Verification items for the finished model (mm, model axes). A direction names the side the tool comes from. Give positions to 0.01 mm unless a question says otherwise; leave off trailing zeros. Order: outer loops, then holes, each group sorted by start corner. A loop starts at its lowest first (then second) coordinate and runs counter-clockwise, first axis right, second up.
(1) Access from +Z, -Z, +X, -X, +Y, -Y to the whole of each face (thin tool, end or side, straight path). Record for faces 4 (the face through (-14.33, -0.37, 1.52)), 5 (the face through (-38.7, -39.23, 1.52)).
(2) Sectioned sample at B-B on x = -7.5. Record the cut outline in (y, z).
(3) Gauge pin test, flat ends, axial feed: pin 1 (4 mm diameter, centred on x = -7.5, y = -65, fed in from +Z); pin 2 (0.9 mm diameter, centred on x = -51.5, z = 1.5, fed in from -Y); pin 3 (1.5 mm diameter, centred on x = -29.5, z = 1, fed in from -Y); pin 4 (0.9 mm diameter, centred on y = -29.5, z = 1.5, fed in from -X). Record the tip position at first contact, or that the pin passes through.
(4) Sectioned sample at A-A on z = 2.45. Count the separate pieces of the cut face and the enclosed holes in it, plus the area to 3 significant figures.
(5) Mould release check, pull along X, two halves, no side actions. Record for faces 1 (the face through (-25.273, -5.418, 1.479)), 2 (the face through (-69, -2, 2)), 3 (the face through (0, -41, 1)): pulls with the +X half, pulls with the -X half, needs draft (parallel to the pull), parting line crosses it, or undercut.
(6) Scan lines: L1, parallel to X at y = -46, z = 1.85; L2, parallel to X at y = -25, z = 0.7; L3, parallel to X at y = -45, z = 1.25. Record each from-to range of solid material in increasing order.
```python
from build123d import *

# Parameters (mm, degrees)
SKETCH_1_R               = 2.1
EXTRUDE_1_DEPTH          = 3
EXTRUDE_2_DEPTH          = 3
CUT_EXTRUDE_1_DEPTH      = 100.040395799
CUT_EXTRUDE_1_DEPTH_BACK = 3
FILLET_1_R               = 5
EXTRUDE_3_DEPTH          = 3
FILLET_2_R               = 3
FILLET_3_R               = 10


with BuildPart() as part:
    # 草图1 → 凸台-拉伸1 (new body)
    with BuildSketch(Plane.XY):
        Polygon((0, 0), (-70, 0), (-70, -15), (-15, -15), (-15, -70), (0, -70), align=None)
        with Locations((-25, -7.5)):
            Circle(SKETCH_1_R, mode=Mode.SUBTRACT)
        with Locations(Location((-7.5, -25, 0), (0, 0, 180))):
            Circle(SKETCH_1_R, mode=Mode.SUBTRACT)
        with Locations((-45, -7.5)):
            Circle(SKETCH_1_R, mode=Mode.SUBTRACT)
        with Locations((-65, -7.5)):
            Circle(SKETCH_1_R, mode=Mode.SUBTRACT)
        with Locations(Location((-7.5, -65, 0), (0, 0, 180))):
            Circle(SKETCH_1_R, mode=Mode.SUBTRACT)
        with Locations(Location((-7.5, -45, 0), (0, 0, 180))):
            Circle(SKETCH_1_R, mode=Mode.SUBTRACT)
    extrude(amount=EXTRUDE_1_DEPTH)

    # 草图2 → 凸台-拉伸2 (add)
    with BuildSketch(Plane.XY.offset(3)):
        Polygon((-70, -15), (-15, -70), (-15, -62.928932188), (-62.928932188, -15), align=None)
    extrude(amount=-EXTRUDE_2_DEPTH)

    # 草图3 → 切除-拉伸1 (cut, two sides: drawn at the far end of the back side and taken through both)
    with BuildSketch(Plane.XY.offset(3).offset(-CUT_EXTRUDE_1_DEPTH_BACK)):
        Polygon((-147.863122604, 133.72098698), (-14.142135624, 0), (0, -14.142135624), (133.72098698, -147.863122604), (401.162960941, 119.578851357), (119.578851357, 401.162960941), align=None)
    extrude(amount=CUT_EXTRUDE_1_DEPTH + CUT_EXTRUDE_1_DEPTH_BACK, mode=Mode.SUBTRACT)

    # 圆角1
    fillet_1_edges = [part.edges().sort_by_distance(p)[0] for p in [
        (0, -70, 1.5),
        (-15, -70, 1.5),
        (-70, -15, 1.5),
        (-70, 0, 1.5),
        (-14.142135624, 0, 1.5),
        (0, -14.142135624, 1.5),
    ]]
    fillet(fillet_1_edges, radius=FILLET_1_R)

    # 草图4 → 凸台-拉伸3 (add, through all)
    with BuildSketch(Plane.XY.offset(3)):
        Polygon((-45.95836944, -15), (-15, -45.95836944), (-15, -38.887301628), (-38.887301628, -15), align=None)
    extrude(amount=-EXTRUDE_3_DEPTH)

    # 圆角2
    fillet_2_edges = [part.edges().sort_by_distance(p)[0] for p in [
        (-45.95836944, -15, 1.5),
        (-38.887301628, -15, 1.5),
        (-15, -38.887301628, 1.5),
        (-15, -45.95836944, 1.5),
        (-62.928932188, -15, 1.5),
        (-15, -62.928932188, 1.5),
    ]]
    fillet(fillet_2_edges, radius=FILLET_2_R)

    # 圆角3
    fillet_3_edges = [part.edges().sort_by_distance(p)[0] for p in [
        (-15, -15, 1.5),
    ]]
    fillet(fillet_3_edges, radius=FILLET_3_R)


solid = part.part
```
Ans:
1. face 4: +Z, -Z, +X, +Y
1. face 5: +Z, -Z
2. outline: (-70, 0) - (-67.1, 0) - (-67.1, 3) - (-70, 3) - close; (-62.9, 0) - (-47.1, 0) - (-47.1, 3) - (-62.9, 3) - close; (-42.9, 0) - (-27.1, 0) - (-27.1, 3) - (-42.9, 3) - close; (-22.9, 0) - (-6.64, 0) - (-6.64, 3) - (-22.9, 3) - close
3. pin 1: passes through
3. pin 2: stops at y = -33.95
3. pin 3: stops at y = -56.25
3. pin 4: stops at x = -55.95
4. separate pieces: 1
4. enclosed holes: 8
4. area: 2,300 mm2
5. face 1: undercut
5. face 2: pulls with the -X half
5. face 3: pulls with the +X half
6. L1: x = -39 to -31.93, -15.25 to -9.35, -5.65 to 0
6. L2: x = -60 to -52.93, -35.96 to -28.89, -15 to -9.6, -5.4 to 0
6. L3: x = -40 to -32.93, -15.96 to -9.6, -5.4 to 0
